Part model, mm, in its own coordinate system. A direction names the side the tool comes from. Give positions to 0.01 mm unless a question says otherwise; leave off trailing zeros. Loops run counter-clockwise (first coordinate to the right, second up) from the corner with the lowest first, then second, coordinate; pieces in that order, holes last. Notation, with made-up numbers: M -7.75,-39.5 L 27.25,-39.5 A32 ccw 27.25,-1.5 Z; hole C 8,55.25 d10. An arc over 180 degrees is marked long. Answer in a Markdown table with one row per item.
from build123d import *

# Parameters (mm, degrees)
ESQUISSE1_W              = 10.2
ESQUISSE1_H              = 15.1
ESQUISSE1_R              = 1.85
BOSS_EXTRU_1_DEPTH       = 1.27
ESQUISSE2_W              = 10.2
ESQUISSE2_H              = 8.6
BOSS_EXTRU_2_DEPTH       = 3.18
ENL_V_MAT_EXTRU_1_DEPTH  = 11.944062317
ENL_V_MAT_EXTRU_2_DEPTH  = 19.757731739
ESQUISSE5_W              = 1.5
ESQUISSE5_H              = 0.5
BOSS_EXTRU_3_DEPTH       = 3.1
ESQUISSE6_W              = 0.8
ESQUISSE6_H              = 0.5
BOSS_EXTRU_4_DEPTH       = 3.5
CHANFREIN1_SIZE          = 0.35
CHANFREIN2_SIZE          = 1
ESQUISSE8_W              = 1.27
ESQUISSE8_H              = 5.5
ENL_V_MAT_EXTRU_4_DEPTH  = 0.01
ESQUISSE9_W              = 1.27
ESQUISSE9_H              = 5.5
ENL_V_MAT_EXTRU_5_DEPTH  = 0.01
BOSS_EXTRU_6_DEPTH       = 0.01
ESQUISSE12_W             = 5.88
ESQUISSE12_H             = 3.15
ENL_V_MAT_EXTRU_15_DEPTH = 17.267993115
BALAYAGE1_START          = -2.94
BALAYAGE1_DEPTH          = 0.8
BALAYAGE2_START          = 2.14
BALAYAGE2_DEPTH          = 0.8
BALAYAGE3_START          = -0.4
BALAYAGE3_DEPTH          = 0.8


# Read off the part's stored shape, not the designer's step: Balayage1, Balayage2, Balayage3
with BuildPart() as part:
    # Esquisse1 → Boss.-Extru.1 (new body)
    with BuildSketch(Plane.XY):
        with Locations((0, 7.55)):
            Rectangle(ESQUISSE1_W, ESQUISSE1_H)
        with Locations((0, 12.36)):
            Circle(ESQUISSE1_R, mode=Mode.SUBTRACT)
    extrude(amount=BOSS_EXTRU_1_DEPTH)

    # Esquisse2 → Boss.-Extru.2 (add)
    with BuildSketch(Plane.XY.offset(1.27)):
        with Locations((0, 4.3)):
            Rectangle(ESQUISSE2_W, ESQUISSE2_H)
    extrude(amount=BOSS_EXTRU_2_DEPTH)

    # Esquisse3 → Enlèv. mat.-Extru.1 (cut, through all)
    with BuildSketch(Plane(origin=(0, 8.6, 0), x_dir=(1, 0, 0), z_dir=(0, 1, 0))):
        Polygon((5.1, -1.27), (4.9, -4.45), (5.1, -4.45), align=None)
        Polygon((-5.1, -1.27), (-5.1, -4.45), (-4.9, -4.45), align=None)
    extrude(amount=-ENL_V_MAT_EXTRU_1_DEPTH, mode=Mode.SUBTRACT)

    # Esquisse4 → Enlèv. mat.-Extru.2 (cut, through all)
    with BuildSketch(Plane(origin=(5.1, 0, 0), x_dir=(0, 0, -1), z_dir=(1, 0, 0))):
        Polygon((-1.27, 8.6), (-4.45, 8.1), (-4.45, 8.6), align=None)
    extrude(amount=-ENL_V_MAT_EXTRU_2_DEPTH, mode=Mode.SUBTRACT)

    # Esquisse5 → Boss.-Extru.3 (add)
    with BuildSketch(Plane.XZ):
        with Locations((0, 3)):
            Rectangle(ESQUISSE5_W, ESQUISSE5_H)
        with Locations((2.54, 3)):
            Rectangle(ESQUISSE5_W, ESQUISSE5_H)
        with Locations((-2.54, 3)):
            Rectangle(ESQUISSE5_W, ESQUISSE5_H)
    extrude(amount=BOSS_EXTRU_3_DEPTH)

    # Esquisse6 → Boss.-Extru.4 (add)
    with BuildSketch(Plane.XZ.offset(3.1)):
        with Locations((-2.54, 3)):
            Rectangle(ESQUISSE6_W, ESQUISSE6_H)
        with Locations((0, 3)):
            Rectangle(ESQUISSE6_W, ESQUISSE6_H)
        with Locations((2.54, 3)):
            Rectangle(ESQUISSE6_W, ESQUISSE6_H)
    extrude(amount=BOSS_EXTRU_4_DEPTH)

    # Chanfrein1
    chanfrein1_edges = [part.edges().sort_by_distance(p)[0] for p in [
        (2.94, -3.1, 3),
        (0.4, -3.1, 3),
        (-2.14, -3.1, 3),
        (2.14, -3.1, 3),
        (-0.4, -3.1, 3),
        (-2.94, -3.1, 3),
    ]]
    chamfer(chanfrein1_edges, length=CHANFREIN1_SIZE - 0.0001)  # a hair under: the kernel refuses the full size

    # Chanfrein2
    chanfrein2_edges = [part.edges().sort_by_distance(p)[0] for p in [
        (-5.1, 15.1, 0.635),
        (5.1, 15.1, 0.635),
    ]]
    chamfer(chanfrein2_edges, length=CHANFREIN2_SIZE)

    # Esquisse8 → Enlèv. mat.-Extru.4 (cut)
    with BuildSketch(Plane(origin=(5.1, 0, 0), x_dir=(0, 0, -1), z_dir=(1, 0, 0))):
        with Locations((-0.635, 11.35)):
            Rectangle(ESQUISSE8_W, ESQUISSE8_H)
    extrude(amount=-ENL_V_MAT_EXTRU_4_DEPTH, mode=Mode.SUBTRACT)

    # Esquisse9 → Enlèv. mat.-Extru.5 (cut)
    with BuildSketch(Plane.ZY.offset(5.1)):
        with Locations((0.635, 11.35)):
            Rectangle(ESQUISSE9_W, ESQUISSE9_H)
    extrude(amount=-ENL_V_MAT_EXTRU_5_DEPTH, mode=Mode.SUBTRACT)

    # Esquisse11 → Boss.-Extru.6 (add)
    with BuildSketch(Plane(origin=(0, 0, 0), x_dir=(-1, 0, 0), z_dir=(0, 0, -1))):
        Polygon((-5.1, 0), (-5.1, 8.6), (-3.6, 8.6), (-3.6, 2), (3.59, 2), (3.59, 8.6), (5.09, 8.6), (5.1, 0), align=None)
    extrude(amount=BOSS_EXTRU_6_DEPTH)

    # Esquisse12 → Enlèv. mat.-Extru.15 (cut, through all)
    with BuildSketch(Plane.XY.offset(3.25)):
        with Locations((0, -5.025)):
            Rectangle(ESQUISSE12_W, ESQUISSE12_H)
    extrude(amount=-ENL_V_MAT_EXTRU_15_DEPTH, mode=Mode.SUBTRACT)

    # Balayage1 outline → Balayage1 (add)
    with BuildSketch(Plane.YZ.offset(BALAYAGE1_START)):
        with BuildLine():
            Line((-4.45, 2.5), (-4.45, -3.51))
            Line((-4.45, -3.51), (-3.95, -3.51))
            Line((-3.95, -3.51), (-3.95, 2.5))
            ThreePointArc((-3.95, 2.5), (-3.876776695, 2.676776695), (-3.7, 2.75))
            Line((-3.7, 2.75), (-3.45, 2.750000001))
            Line((-3.45, 2.750000001), (-3.45, 3.25))
            Line((-3.45, 3.25), (-3.7, 3.25))
            ThreePointArc((-3.7, 3.25), (-4.230330086, 3.030330086), (-4.45, 2.5))
        make_face()
    extrude(amount=BALAYAGE1_DEPTH)

    # Balayage2 outline → Balayage2 (add)
    with BuildSketch(Plane.YZ.offset(BALAYAGE2_START)):
        with BuildLine():
            Line((-4.45, 2.5), (-4.45, -3.51))
            Line((-4.45, -3.51), (-3.95, -3.51))
            Line((-3.95, -3.51), (-3.95, 2.5))
            ThreePointArc((-3.95, 2.5), (-3.876776695, 2.676776695), (-3.7, 2.75))
            Line((-3.7, 2.75), (-3.45, 2.750000001))
            Line((-3.45, 2.750000001), (-3.45, 3.25))
            Line((-3.45, 3.25), (-3.7, 3.25))
            ThreePointArc((-3.7, 3.25), (-4.230330086, 3.030330086), (-4.45, 2.5))
        make_face()
    extrude(amount=BALAYAGE2_DEPTH)

    # Balayage3 outline → Balayage3 (add)
    with BuildSketch(Plane.YZ.offset(BALAYAGE3_START)):
        with BuildLine():
            Line((-4.45, 2.5), (-4.45, -3.51))
            Line((-4.45, -3.51), (-3.95, -3.51))
            Line((-3.95, -3.51), (-3.95, 2.5))
            ThreePointArc((-3.95, 2.5), (-3.876776695, 2.676776695), (-3.7, 2.75))
            Line((-3.7, 2.75), (-3.45, 2.750000001))
            Line((-3.45, 2.750000001), (-3.45, 3.25))
            Line((-3.45, 3.25), (-3.7, 3.25))
            ThreePointArc((-3.7, 3.25), (-4.230330086, 3.030330086), (-4.45, 2.5))
        make_face()
    extrude(amount=BALAYAGE3_DEPTH)


solid = part.part
(1) Pin check, flat tips, straight feed: pin 1 Ø0.8 at (y, z) = (-4, 1.5) entering from -X; pin 2 Ø3 at (x, y) = (0, 12.36) entering from +Z; pin 3 Ø1.4 at (y, z) = (11.5, 1) entering from +X; pin 4 Ø5 at (x, y) = (2, 13.5) entering from +Z. Stop position of each tip, or through.
Recorded:
| item | result |
|---|---|
| pin 1 | stops at x = -2.94 |
| pin 2 | passes through |
| pin 3 | stops at x = 5.09 |
| pin 4 | stops at z = 1.27 |
(2) Saw through at A-A (z = 0.25). Give the number of separate pieces and of enclosed holes in the cut face, plus the area to 3 significant figures.
Recorded:
| item | result |
|---|---|
| separate pieces | 4 |
| enclosed holes | 1 |
| area | 143 mm^2 |
(3) Pull direction X, two halves, no side cores. Call faces 6 (the face through (-0.4, -4.2, -0.1)), 7 (the face through (-5.1, 4, 1)), 8 (the face through (0, 1, -0.01)), 9 (the face through (5, 4.36, 2.84)): +X half, -X half, draft (parallel to the pull), parting line (faces both ways), or undercut.
Recorded:
| item | result |
|---|---|
| face 6 | undercut |
| face 7 | -X half |
| face 8 | draft |
| face 9 | +X half |
(4) Saw through at C-C (z = -1.25). Write the cut outline in (x, y).
Recorded:
| item | result |
|---|---|
| outline | M -2.94,-4.45 L -2.14,-4.45 L -2.14,-3.95 L -2.94,-3.95 Z; M -0.4,-4.45 L 0.4,-4.45 L 0.4,-3.95 L -0.4,-3.95 Z; M 2.14,-4.45 L 2.94,-4.45 L 2.94,-3.95 L 2.14,-3.95 Z |
(5) Saw through at B-B (y = 12.36). Write the cut outline in (x, z).
Recorded:
| item | result |
|---|---|
| outline | M -5.09,0 L -1.85,0 L -1.85,1.27 L -5.09,1.27 Z; M 1.85,0 L 5.09,0 L 5.09,1.27 L 1.85,1.27 Z |
(6) Which spindle directions (+Z, -Z, +X, -X, +Y, -Y) get a long thin tool onto all of the face, cutting with end or side? Do faces 1 (the face through (-2.94, -4.2, -0.1)), 2 (the face through (0, 15.1, 1)), 3 (the face through (3, -2, 3.25)), 4 (the face through (2.14, -4.2, -0.1)), 5 (the face through (0, 10, 1.27)). Say none if no direction does.
Recorded:
| item | result |
|---|---|
| face 1 | +Z, -Z, -X, -Y |
| face 2 | +Z, -Z, +X, -X, +Y |
| face 3 | +Z, +X, -X, -Y |
| face 4 | +Z, -Z, -Y |
| face 5 | +Z, +X, -X, +Y |
(7) Drill centre lines: line 1 along Y through (x, z) = (0, 0.35); line 2 along Z through (x, y) = (0.5, 2); line 3 along Z through (x, y) = (-2.25, 9.5). Where is each one in solid material? Low to high.
Recorded:
| item | result |
|---|---|
| line 1 | y = -4.45 to -3.95, 0 to 10.51, 14.21 to 15.1 |
| line 2 | z = 0 to 4.45 |
| line 3 | z = 0 to 1.27 |
